Source: CAD feature listing. Evaluate the final solid. Frame: model axes, mm. Round coordinates to 2 decimals unless told otherwise and drop trailing zeros. Write each loop counter-clockwise with the first axis right and the second up, starting at its lowest first coordinate (ties: lowest second). Pieces come first, ordered by that corner, then holes. Notation, with made-up numbers: (-13.5, 24.5) -> (37.5, 24.5) arc R26 ccw to (37.5, 51.5) -> close; hole circle Ø11 at (22, 61.5). An arc over 180 degrees is marked (long way). Return JSON: item names as keys, results as strings. Group by question number.
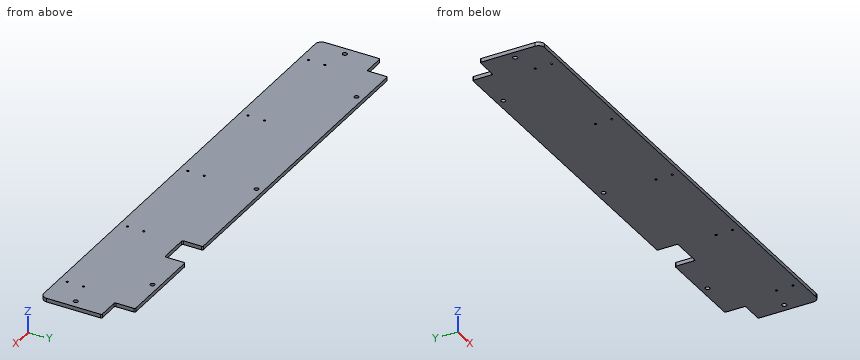
Autodesk Inventor part; units mm, degrees
ref_plane "YZ Plane" through (0, 0, 0) normal (1, 0, 0) x (0, 1, 0)
ref_plane "XZ Plane" through (0, 0, 0) normal (0, 1, 0) x (-1, 0, 0)
ref_plane "XY Plane" through (0, 0, 0) normal (0, 0, 1) x (1, 0, 0)
sketch "Sketch1" plane through (0, 0, 0) normal (0, 0, 1) x (1, 0, 0)
  line L0 (0, 88.9) -> (0, -88.9)
  line L1 (-533.4, 0) -> (533.4, 0)
  line L2 (381, -63.5) -> (-381, -63.5)
  line L3 (-381, -63.5) -> (-381, 63.5)
  line L4 (-381, 63.5) -> (381, 63.5)
  line L5 (381, 63.5) -> (381, -63.5)
  line L6 (381, -63.5) -> (-381, 63.5) construction
  line L7 (-381, -63.5) -> (381, 63.5) construction
  line L8 (-170.942, -37.592) -> (-127, -37.592) construction
  line L9 (-127, -37.592) -> (-127, -63.5) construction
  line L10 (-127, -63.5) -> (-170.942, -63.5) construction
  line L11 (-170.942, -63.5) -> (-170.942, -37.592) construction
  line L12 (127, -37.592) -> (170.942, -37.592) construction
  line L13 (170.942, -37.592) -> (170.942, -63.5) construction
  line L14 (170.942, -63.5) -> (127, -63.5) construction
  line L15 (127, -63.5) -> (127, -37.592) construction
  line L16 (-381, 31.75) -> (-345.44, 31.75)
  line L17 (-345.44, 31.75) -> (-345.44, 63.5)
  line L18 (345.44, 63.5) -> (345.44, 31.75)
  line L19 (345.44, 31.75) -> (381, 31.75)
  line L20 (368.3, -44.45) -> (-368.3, -44.45) construction
  line L21 (-368.3, -44.45) -> (-368.3, 12.7) construction
  line L22 (-368.3, 12.7) -> (368.3, 12.7) construction
  line L23 (368.3, 12.7) -> (368.3, -44.45) construction
  line L24 (368.3, -44.45) -> (-368.3, 12.7) construction
  line L25 (-368.3, -44.45) -> (368.3, 12.7) construction
  line L26 (328.6125, -23.8125) -> (357.1875, -23.8125)
  line L27 (357.1875, -23.8125) -> (357.1875, 23.8125)
  line L28 (357.1875, 23.8125) -> (328.6125, 23.8125)
  line L29 (328.6125, 23.8125) -> (328.6125, -23.8125)
  line L30 (328.6125, -23.8125) -> (357.1875, 23.8125) construction
  line L31 (357.1875, -23.8125) -> (328.6125, 23.8125) construction
  line L32 (-42.8625, -23.8125) -> (-14.2875, -23.8125)
  line L33 (-14.2875, -23.8125) -> (-14.2875, 23.8125)
  line L34 (-14.2875, 23.8125) -> (-42.8625, 23.8125)
  line L35 (-42.8625, 23.8125) -> (-42.8625, -23.8125)
  line L36 (-42.8625, -23.8125) -> (-14.2875, 23.8125) construction
  line L37 (-14.2875, -23.8125) -> (-42.8625, 23.8125) construction
  point P0 (0, 0)
  point P1 (-159.004, -63.5)
  point P2 (138.938, -63.5)
  point P3 (-279.4, 53.009)
  point P4 (279.4, 53.009)
  point P5 (-5.08, 53.009)
  point P6 (0, -15.875)
  point P7 (342.9, 0)
  point P8 (-28.575, 0)
  point P9 (-368.3, -15.875)
  point P10 (368.3, -15.875)
  dimension "d0" = 762
  dimension "d1" = 127
  dimension "d2" = 43.942
  dimension "d3" = 25.908
  dimension "d4" = 32.004
  dimension "d5" = 127
  dimension "d7" = 32.004
  dimension "d8" = 127
  dimension "d9" = 10.491
  dimension "d65" = 31.75
  dimension "d66" = 345.44
  dimension "d67" = 736.6
  dimension "d68" = 19.05
  dimension "d69" = 19.05
  dimension "d84" = 279.4
  dimension "d85" = 279.4
  dimension "d86" = 5.08
  dimension "d87" = 28.575
  dimension "d88" = 47.625
  dimension "d89" = 0
  dimension "d90" = 28.575
  dimension "d91" = 342.9
  dimension "d94" = 101.092
extrude "Extrusion1" add sketch "Sketch1" against normal blind 5.842 contours L4 L18 L19 L5 L1 L27 L28 L29 L0 | L0 L1 L33 L34 L35 L3 L16 L17 L4 | L1 L29 L26 L27 L5 L2 L0 | L0 L2 L3 L1 L35 L32 L33 | L33 L32 L35 L1 | L1 L35 L34 L33 | L29 L28 L27 L1 | L1 L27 L26 L29
hole "Hole2" at (-279.4, 53.009, 0) at (279.4, 53.009, 0) at (-5.08, 53.009, 0) direction (0, 0, -1) diameter 6.731 end through all
fillet "Fillet1" radius 9.525 2 edges at (381, -63.5, -2.921) (-381, -63.5, -2.921)
hole "Hole5" at (-368.3, -15.875, 0) at (368.3, -15.875, 0) direction (0, 0, -1) diameter 7.0104 end through all
fillet "Fillet2" radius 1.905 6 edges at (-381, 31.75, -2.921) (-345.44, 31.75, -2.921) (-345.44, 63.5, -2.921) (345.44, 63.5, -2.921) (381, 31.75, -2.921) (345.44, 31.75, -2.921)
sketch "Sketch4" plane through (0, 0, 0) normal (0, 0, 1) x (1, 0, 0)
  line L0 (343.535, 63.5) -> (-343.535, 63.5)
  line L1 (208.5594, 31.75) -> (160.2994, 31.75)
  line L2 (160.2994, 31.75) -> (160.2994, 63.5)
  line L3 (160.2994, 63.5) -> (208.5594, 63.5)
  line L4 (208.5594, 63.5) -> (208.5594, 31.75)
  line L5 (208.5594, 31.75) -> (160.2994, 63.5) construction
  line L6 (160.2994, 31.75) -> (208.5594, 63.5) construction
  line L7 (0, 88.9) -> (0, -88.9)
  point P0 (0, 0)
  point P1 (184.4294, 47.625)
  point P2 (208.5594, 63.5)
  dimension "d78" = 48.26
  dimension "d80" = 31.75
  dimension "d83" = 184.4294
extrude "Extrusion2" cut sketch "Sketch4" against normal through all
fillet "Fillet3" radius 1.905 4 edges at (160.2994, 63.5, -2.921) (160.2994, 31.75, -2.921) (208.5594, 31.75, -2.921) (208.5594, 63.5, -2.921)
sketch "Sketch5" plane through (0, 0, 0) normal (0, 0, 1) x (1, 0, 0)
  line L0 (371.475, -63.5) -> (-371.475, -63.5)
  line L1 (0, 88.9) -> (0, -88.9)
  line L2 (330.2, -50.8) -> (-330.2, -50.8) construction
  line L3 (-371.475, -63.5) -> (371.475, -63.5) construction
  point P0 (0, 0)
  point P1 (0, -50.8)
  point P2 (165.1, -50.8)
  point P3 (-165.1, -50.8)
  dimension "d108" = 330.2
  dimension "d109" = 330.2
  dimension "d110" = 12.7
  dimension "d118" = 165.1
  dimension "d119" = 165.1
hole "Hole6" at (330.2, -50.8, 0) at (0, -50.8, 0) at (-330.2, -50.8, 0) at (165.1, -50.8, 0) at (-165.1, -50.8, 0) direction (0, 0, -1) diameter 3.1242 end through all
pattern_linear "Rectangular Pattern2" count 2 spacing 25.4 along (0, 1, 0) of "Hole6"
properties material "ACRYLIC, BLACK"
Item 1: First-contact query: pin 1 Ø2 at (y, z) = (39.5, -4) entering from +X; pin 2 Ø1 at (y, z) = (33.5, -5) entering from +X; pin 3 Ø3 at (y, z) = (54.5, -4) entering from -X; pin 4 Ø4 at (x, y) = (330.2, -25.4) entering from -Z. Flat tips, straight axial feed; report the tip coordinate or a pass-through.
Item 2: Cut plane A-A on y = 41.5. Output: boundary loops of the cut face in (x, z).
Item 3: Cut plane B-B on z = -4.8. Give the number of separate pieces and of enclosed holes in the cut face, and give its area (3 significant figures).
Item 4: Material intervals for probe 1 along X at (y, z) = (53, -2.5); probe 2 along Y at (x, z) = (-165.1, -4); probe 3 along X at (y, z) = (-50.8, -1.75), sorted ascending.
Here are the results:
{
 "1": {"pin 1": "stops at x = 345.44", "pin 2": "stops at x = 345.56", "pin 3": "stops at x = -345.44", "pin 4": "stops at z = -5.84"},
 "2": {"outline": "(-345.44, -5.84) -> (160.3, -5.84) -> (160.3, 0) -> (-345.44, 0) -> close; (208.56, -5.84) -> (345.44, -5.84) -> (345.44, 0) -> (208.56, 0) -> close"},
 "3": {"separate pieces": "1", "enclosed holes": "15", "area": "92,700 mm^2"},
 "4": {"probe 1": "x = -345.44 to -282.77, -276.03 to -8.45, -1.71 to 160.3, 208.56 to 276.03, 282.77 to 345.44", "probe 2": "y = -63.5 to -52.36, -49.24 to -26.96, -23.84 to 63.5", "probe 3": "x = -381 to -331.76, -328.64 to -166.66, -163.54 to -1.56, 1.56 to 163.54, 166.66 to 328.64, 331.76 to 381"}
}
